from build123d import *

# Parameters (mm, degrees)
SKETCH1_R           = 17.5
SKETCH1_R_2         = 1.5
BOSS_EXTRUDE1_DEPTH = 5
SKETCH2_R           = 3.25
CUT_EXTRUDE1_DEPTH  = 1.5


with BuildPart() as part:
    # Sketch1 → Boss-Extrude1 (new body)
    with BuildSketch(Plane(origin=(0, 0, 0), x_dir=(1, 0, 0), z_dir=(0, 1, 0))):
        with Locations(Location((0, 0, 0), (0, 0, 270))):
            Circle(SKETCH1_R)
        with Locations(Location((0, 14, 0), (0, 0, 270))):
            Circle(SKETCH1_R_2, mode=Mode.SUBTRACT)
        with Locations(Location((12.124355653, 7, 0), (0, 0, 270))):
            Circle(SKETCH1_R_2, mode=Mode.SUBTRACT)
        with Locations(Location((12.124355653, -7, 0), (0, 0, 270))):
            Circle(SKETCH1_R_2, mode=Mode.SUBTRACT)
        with Locations(Location((0, -14, 0), (0, 0, 270))):
            Circle(SKETCH1_R_2, mode=Mode.SUBTRACT)
        with Locations(Location((-12.124355653, -7, 0), (0, 0, 270))):
            Circle(SKETCH1_R_2, mode=Mode.SUBTRACT)
        with Locations(Location((-12.124355653, 7, 0), (0, 0, 270))):
            Circle(SKETCH1_R_2, mode=Mode.SUBTRACT)
        Polygon((7.505553499, 0), (3.75277675, 6.5), (-3.75277675, 6.5), (-7.505553499, 0), (-3.75277675, -6.5), (3.75277675, -6.5), align=None, mode=Mode.SUBTRACT)
    extrude(amount=BOSS_EXTRUDE1_DEPTH)

    # Sketch2 → Cut-Extrude1 (cut)
    with BuildSketch(Plane(origin=(0, 5, 0), x_dir=(1, 0, 0), z_dir=(0, 1, 0))):
        with Locations(Location((0, 14, 0), (0, 0, 270))):
            Circle(SKETCH2_R)
        with Locations(Location((12.124355653, 7, 0), (0, 0, 270))):
            Circle(SKETCH2_R)
        with Locations(Location((12.124355653, -7, 0), (0, 0, 270))):
            Circle(SKETCH2_R)
        with Locations(Location((0, -14, 0), (0, 0, 270))):
            Circle(SKETCH2_R)
        with Locations(Location((-12.124355653, -7, 0), (0, 0, 270))):
            Circle(SKETCH2_R)
        with Locations(Location((-12.124355653, 7, 0), (0, 0, 270))):
            Circle(SKETCH2_R)
    extrude(amount=-CUT_EXTRUDE1_DEPTH, mode=Mode.SUBTRACT)


solid = part.part
Could you check a few things on this model? Use its own coordinates, in mm. A direction names the side the tool comes from. Give positions to 0.01 mm unless a question says otherwise; leave off trailing zeros. Write each loop counter-clockwise with the first axis right and the second up, starting at its lowest first coordinate (ties: lowest second). Pieces come first, ordered by that corner, then holes. Notation, with made-up numbers: (10.5, 21) -> (28.5, 21) arc R13 ccw to (28.5, 43) -> close; hole circle Ø8 at (-12, 81). An arc over 180 degrees is marked (long way). Answer as CSV lines item,"result". Start each with the question number.
(1) If we mould it in two halves opening along X, with no side actions, what happens to faces 1 (the face through (0, 2, 6.5)), 2 (the face through (-10.648, 2.465, -13.887)), 3 (the face through (0, 5, 8))? For each: +X half, -X half, draft (parallel to the pull), parting line (faces both ways), or undercut.
(2) If we section it at C-C, the plane x = -5: Write out the boundary of the cut face in (y, z).
(3) Which directions (+Z, -Z, +X, -X, +Y, -Y) give clear straight access to the entire face, cutting with the end or side of a thin tool? Please do faces 4 (the face through (11.4, 3.5, -8.5)), 5 (the face through (5.66, 2.46, -3.2)).
(4) If we section it at D-D, the plane y = 4.45: Write out the boundary of the cut face in (x, z), and give its area (3 significant figures).
(5) If we section it at B-B, the plane z = 14: Write out the boundary of the cut face in (x, y).
(6) Please list where these lines run through material, in increasing order: line 1 (X direction, y = 4, z = -7); line 2 (X direction, y = 3.65, z = 8.5); line 3 (Z direction, x = -9.5, y = 4.85).
(7) If we section it at A-A, the plane x = 0: Write out the boundary of the cut face in (y, z).
(8) I'm going to push flat-ended pins straight in: pin 1 Ø2 at (x, z) = (13, 6) entering from +Y; pin 2 Ø2.5 at (x, z) = (-12.12, -7) entering from +Y; pin 3 Ø3 at (y, z) = (3, -2.5) entering from +X. Where does each tip first touch, or does it pass through?
Answer list:
1,face 1,"undercut"
1,face 2,"parting line"
1,face 3,"draft"
2,outline,"(0, -16.77) -> (5, -16.77) -> (5, -4.34) -> (0, -4.34) -> close; (0, 4.34) -> (5, 4.34) -> (5, 16.77) -> (0, 16.77) -> close"
3,face 4,"+Y"
3,face 5,"+Y, -Y"
4,outline,"circle Ø35 at (0, 0); hole circle Ø6.5 at (-12.12, -7); hole circle Ø6.5 at (-12.12, 7); hole (-7.51, 0) -> (-3.75, -6.5) -> (3.75, -6.5) -> (7.51, 0) -> (3.75, 6.5) -> (-3.75, 6.5) -> close; hole circle Ø6.5 at (0, -14); hole circle Ø6.5 at (0, 14); hole circle Ø6.5 at (12.12, -7); hole circle Ø6.5 at (12.12, 7)"
4,area,"617 mm^2"
5,outline,"(-10.5, 0) -> (-1.5, 0) -> (-1.5, 3.5) -> (-3.25, 3.5) -> (-3.25, 5) -> (-10.5, 5) -> close; (1.5, 0) -> (10.5, 0) -> (10.5, 5) -> (3.25, 5) -> (3.25, 3.5) -> (1.5, 3.5) -> close"
6,line 1,"-16.04 to -15.37, -8.87 to 8.87, 15.37 to 16.04"
6,line 2,"-15.3 to -15.01, -9.24 to 9.24, 15.01 to 15.3"
6,line 3,"-14.7 to -8.92, -5.08 to 5.08, 8.92 to 14.7"
7,outline,"(0, -17.5) -> (5, -17.5) -> (5, -17.25) -> (3.5, -17.25) -> (3.5, -15.5) -> (0, -15.5) -> close; (0, -12.5) -> (3.5, -12.5) -> (3.5, -10.75) -> (5, -10.75) -> (5, -6.5) -> (0, -6.5) -> close; (0, 6.5) -> (5, 6.5) -> (5, 10.75) -> (3.5, 10.75) -> (3.5, 12.5) -> (0, 12.5) -> close; (0, 15.5) -> (3.5, 15.5) -> (3.5, 17.25) -> (5, 17.25) -> (5, 17.5) -> (0, 17.5) -> close"
8,pin 1,"y = 3.5"
8,pin 2,"through"
8,pin 3,"x = 17.47"
